Geometry check sheet. Reference: the model listing, model coordinates, mm. A direction names the side the tool comes from. Give positions to 0.01 mm unless a question says otherwise; leave off trailing zeros. Loops run counter-clockwise (first coordinate to the right, second up) from the corner with the lowest first, then second, coordinate; pieces in that order, holes last. Notation, with made-up numbers: (4.25, 56.5) -> (40.25, 56.5) arc R18 cw to (40.25, 83.5) -> close; hole circle Ø11 at (40, 2.25). An arc over 180 degrees is marked (long way). Write item = value, one per line.
```python
from build123d import *

# Parameters (mm, degrees)
SKETCH1_R           = 10
BOSS_EXTRUDE1_DEPTH = 50
SKETCH7_R           = 10
SKETCH7_R_2         = 9.5
CUT_EXTRUDE1_DEPTH  = 10
SKETCH10_W          = 2.65
SKETCH10_H          = 10
SKETCH11_R          = 11
BOSS_EXTRUDE2_DEPTH = 3


# Read off the part's stored shape, not the designer's step: M18x2.5 Machine Threads Stud1, M18x2.5 Machine Threads Stud2
with BuildPart() as part:
    # Sketch1 → Boss-Extrude1 (new, symmetric)
    with BuildSketch(Plane.XY):
        Circle(SKETCH1_R)
    extrude(amount=BOSS_EXTRUDE1_DEPTH, both=True)

    # M18x2.5 Machine Threads Stud1 outline → M18x2.5 Machine Threads Stud1 (revolve, cut)
    with BuildSketch(Plane.XZ):
        Polygon((7.626, -50), (10, -50), (10, -35), (9, -35), (9, -48.626), align=None)
    revolve(axis=Axis((0, 0, 0), (0, 0, 1)), mode=Mode.SUBTRACT)

    # M18x2.5 Machine Threads Stud2 outline → M18x2.5 Machine Threads Stud2 (revolve, cut)
    with BuildSketch(Plane.XZ):
        Polygon((10, 50), (7.626, 50), (9, 48.626), (9, 35), (10, 35), align=None)
    revolve(axis=Axis((0, 0, 0), (0, 0, 1)), mode=Mode.SUBTRACT)

    # Sketch7 → Cut-Extrude1 (cut)
    with BuildSketch(Plane.XY.offset(35)):
        Circle(SKETCH7_R)
        Circle(SKETCH7_R_2, mode=Mode.SUBTRACT)
    extrude(amount=-CUT_EXTRUDE1_DEPTH, mode=Mode.SUBTRACT)

    # Sketch10 → M5 Clearance Hole1 (revolve, cut)
    with BuildSketch(Plane(origin=(0, 0, 30), x_dir=(0, 0, -1), z_dir=(1, 0, 0))):
        with Locations((1.325, 5)):
            Rectangle(SKETCH10_W, SKETCH10_H)
    m5_clearance_hole1 = revolve(axis=Axis((0, -6.35, 30), (0, 1, 0)), mode=Mode.SUBTRACT)

    # Mirror2: M5 Clearance Hole1 across plane
    add(m5_clearance_hole1.mirror(Plane.ZX), mode=Mode.SUBTRACT)

    # Sketch11 → Boss-Extrude2 (add)
    with BuildSketch(Plane.XY.offset(25)):
        Circle(SKETCH11_R)
    extrude(amount=-BOSS_EXTRUDE2_DEPTH)


solid = part.part
```
Item 1: Tool access check on faces 4 (the flat face through (-9, 2, -35)), 5 (the flat face through (-10, 0, 25)), 6 (the flat face through (0, 0, 50)). Record the directions out of +Z, -Z, +X, -X, +Y, -Y that give a thin tool (end or side, any length) a straight path to the whole face; none if there is none.
Answer:
face_4 = -Z
face_5 = +Z
face_6 = +Z, +X, -X, +Y, -Y
Item 2: Section check C-C, the plane z = 43. Record the cut outline in (x, y).
Answer:
outline = circle Ø18 at (0, 0)
Item 3: Draft check along X on faces 1 (the cylindrical face through (-0.117, 0.133, 32.647)), 2 (the flat face through (0, 0, -50)), 3 (the cylindrical face through (-2.17, -9.76, -6.1)). Enter one of: +X half, -X half, draft (parallel to the pull), parting line (faces both ways), or undercut.
Answer:
face_1 = undercut
face_2 = draft
face_3 = parting line
Item 4: Section check A-A, the plane x = 0. Record the cut outline in (y, z).
Answer:
outline = (-11, 22) -> (-10, 22) -> (-10, -35) -> (-9, -35) -> (-9, -48.63) -> (-7.63, -50) -> (7.63, -50) -> (9, -48.63) -> (9, -35) -> (10, -35) -> (10, 22) -> (11, 22) -> (11, 25) -> (9.5, 25) -> (9.5, 27.35) -> (-9.5, 27.35) -> (-9.5, 25) -> (-11, 25) -> close; (-9.5, 32.65) -> (9.5, 32.65) -> (9.5, 35) -> (9, 35) -> (9, 48.63) -> (7.63, 50) -> (-7.63, 50) -> (-9, 48.63) -> (-9, 35) -> (-9.5, 35) -> close
Item 5: Gauge pin test, flat ends, axial feed: pin 1 (5 mm diameter, centred on x = -3.5, z = 35, fed in from -Y); pin 2 (3 mm diameter, centred on x = 6.5, z = -30, fed in from -Y); pin 3 (1 mm diameter, centred on x = 0, z = 13.5, fed in from +Y). Record the tip position at first contact, or that the pin passes through.
Answer:
pin_1 = -9.45
pin_2 = -8.66
pin_3 = 10
Item 6: Section check B-B, the plane y = 0. Record the cut outline in (x, z).
Answer:
outline = (-11, 22) -> (-10, 22) -> (-10, -35) -> (-9, -35) -> (-9, -48.63) -> (-7.63, -50) -> (7.63, -50) -> (9, -48.63) -> (9, -35) -> (10, -35) -> (10, 22) -> (11, 22) -> (11, 25) -> (9.5, 25) -> (9.5, 35) -> (9, 35) -> (9, 48.63) -> (7.63, 50) -> (-7.63, 50) -> (-9, 48.63) -> (-9, 35) -> (-9.5, 35) -> (-9.5, 25) -> (-11, 25) -> close; hole circle Ø5.3 at (0, 30)
Item 7: Section check D-D, the plane z = 30. Record the cut outline in (x, y).
Answer:
outline = (-2.65, -9.12) -> (-2.65, 9.12) arc R9.5 ccw to start; (2.65, -9.12) arc R9.5 ccw to (2.65, 9.12) -> close
Item 8: Thickness scan on L1, parallel to Z at x = 0, y = 5.25; L2, parallel to Z at x = 0.5, y = 10.25; L3, parallel to Y at x = 0, z = 18. Record the ranges inside material, lowest first. Write a range as [from, to].
Answer:
L1 = [-50, 27.35], [32.65, 50]
L2 = [22, 25]
L3 = [-10, 10]
